```python
from build123d import *

# Parameters (mm, degrees)
EXTRUDE_1_DEPTH              = 5
SKETCH_2_R                   = 6.25
EXTRUDE_2_DEPTH              = 3
SKETCH_3_R                   = 5
EXTRUDE_3_DEPTH              = 5
HOLE_WIZARD_M4_1_D           = 4.5
HOLE_WIZARD_M4_1_CBORE_D     = 9
HOLE_WIZARD_M4_1_CBORE_DEPTH = 4
EXTRUDE_4_DEPTH              = 5
EXTRUDE_5_DEPTH              = 5
EXTRUDE_5_DEPTH_BACK         = 5
EXTRUDE_6_DEPTH              = 4.5
SKETCH_15_R                  = 10
CUT_EXTRUDE_2_DEPTH          = 20


with BuildPart() as part:
    # Sketch 1 → Extrude 1 (new body)
    with BuildSketch(Plane(origin=(0, 0, 0), x_dir=(1, 0, 0), z_dir=(0, 1, 0))):
        with BuildLine():
            Line((-15, 0), (-15, 60))
            ThreePointArc((-15, 60), (0, 75), (15, 60))
            Line((15, 60), (15, 0))
            ThreePointArc((15, 0), (0, -15), (-15, 0))
        make_face()
    extrude(amount=EXTRUDE_1_DEPTH)

    # Sketch 2 → Extrude 2 (add)
    with BuildSketch(Plane(origin=(0, 5, 0), x_dir=(1, 0, 0), z_dir=(0, 1, 0))):
        with Locations((0, 60)):
            Circle(SKETCH_2_R)
        Circle(SKETCH_2_R)
    extrude(amount=EXTRUDE_2_DEPTH)

    # Sketch 3 → Extrude 3 (add)
    with BuildSketch(Plane(origin=(0, 8, 0), x_dir=(1, 0, 0), z_dir=(0, 1, 0))):
        with Locations((0, 60)):
            Circle(SKETCH_3_R)
        Circle(SKETCH_3_R)
    extrude(amount=EXTRUDE_3_DEPTH)

    # Hole Wizard M4 _ _ _ _1 (through all)
    with Locations(Plane(origin=(0, 0, 0), x_dir=(-1, 0, 0), z_dir=(0, -1, 0))):
        with Locations((0, 60), (0, -25)):
            CounterBoreHole(HOLE_WIZARD_M4_1_D / 2, HOLE_WIZARD_M4_1_CBORE_D / 2, HOLE_WIZARD_M4_1_CBORE_DEPTH)

    # Sketch 8 → Extrude 4 (add)
    with BuildSketch(Plane.XZ):
        with BuildLine():
            Line((-5.13030215, 14.095389312), (23.060476474, 24.355993612))
            ThreePointArc((23.060476474, 24.355993612), (42.286167935, 15.39090645), (33.321080773, -3.834785012))
            Line((33.321080773, -3.834785012), (15, -10.503113073))
            Line((15, -10.503113073), (15, 0))
            ThreePointArc((15, 0), (8.603646545, 12.287280664), (-5.13030215, 14.095389312))
        make_face()
    extrude(amount=-EXTRUDE_4_DEPTH)

    # Sketch 9 → Extrude 5 (add, two sides)
    with BuildSketch(Plane.XZ) as extrude_5_sk:
        with BuildLine():
            Line((14.095389312, 5.13030215), (3.834785012, 33.321080773))
            Line((3.834785012, 33.321080773), (-1.295517138, 47.416470085))
            Line((-1.295517138, 47.416470085), (26.895261486, 57.677074385))
            Line((26.895261486, 57.677074385), (32.025563636, 43.581685073))
            Line((32.025563636, 43.581685073), (42.286167935, 15.39090645))
            ThreePointArc((42.286167935, 15.39090645), (33.321080773, -3.834785012), (14.095389312, 5.13030215))
        make_face()
    extrude(amount=EXTRUDE_5_DEPTH)
    extrude(extrude_5_sk.sketch, amount=-EXTRUDE_5_DEPTH_BACK)

    # Sketch 13 → Extrude 6 (add)
    with BuildSketch(Plane(origin=(0, 5, 0), x_dir=(1, 0, 0), z_dir=(0, 1, 0))):
        Polygon((37.155865785, -29.486295761), (26.895261486, -57.677074385), (-1.295517138, -47.416470085), (8.965087162, -19.225691462), align=None)
    extrude(amount=EXTRUDE_6_DEPTH)

    # Sketch 15 → Cut-Extrude 2 (cut)
    with BuildSketch(Plane(origin=(-15.39090645, 0, 42.286167935), x_dir=(0.939692621, 0, 0.342020143), z_dir=(-0.342020143, 0, 0.939692621))):
        with Locations((30, 10.5)):
            Circle(SKETCH_15_R)
    extrude(amount=-CUT_EXTRUDE_2_DEPTH, mode=Mode.SUBTRACT)


solid = part.part
```
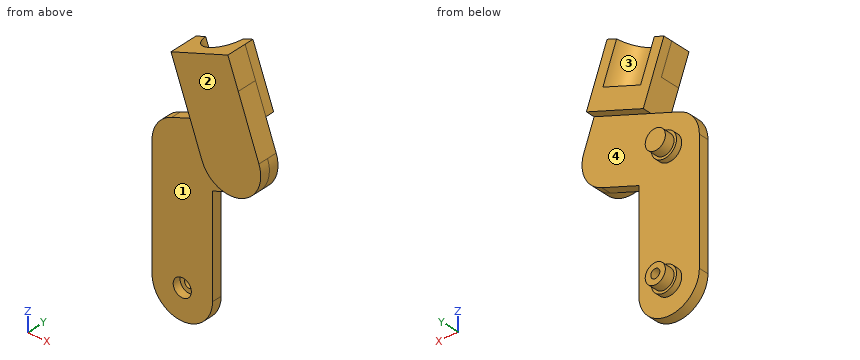
The model under review builds one solid part; all positions refer to its coordinate system, in mm. Face numbers are marked on the shaded views. A direction names the side the tool comes from. Coordinates: 2 decimals unless noted, no trailing zeros. Loops run counter-clockwise (first coordinate to the right, second up) from the corner with the lowest first, then second, coordinate; pieces in that order, holes last. Notation, with made-up numbers: (66.25, 43.25) -> (93.25, 43.25) arc R25 cw to (93.25, 66.25) -> close; hole circle Ø9 at (-5.5, 63). An arc over 180 degrees is marked (long way). Answer as CSV lines item,"result".
Item 1: For L1, parallel to X at y = 10.75, z = -60; L2, parallel to X at y = 2.45, z = -60; L3, parallel to Y at x = -10.5, z = 0, list the stretches that pass through material, from the lowest coordinate up.
Results below:
L1,"x = -5 to -2.25, 2.25 to 5"
L2,"x = -15 to -4.5, 4.5 to 15"
L3,"y = 0 to 5"
Item 2: Take a section at B-B, the plane x = 0. Count the separate pieces of the cut face and the enclosed holes in it, and give its area (3 significant figures).
Results below:
separate pieces,"3"
enclosed holes,"0"
area,"612 mm2"
Item 3: Draft analysis for pull direction X (two halves, no side actions). For the marked faces 3 and 4, state which applies: +X half, -X half, draft (parallel to the pull), parting line (faces both ways), or undercut.
Results below:
face 3,"undercut"
face 4,"draft"
Item 4: Insertion check: pin 1 (4 mm diameter, centred on y = 2, z = -36.5, fed in from +X); pin 2 (7 mm diameter, centred on x = 1.5, z = -59.5, fed in from -Y); pin 3 (3 mm diameter, centred on x = -7, z = -33.5, fed in from +Y); pin 4 (4 mm diameter, centred on x = 0, z = -60, fed in from -Y). Each pin has a flat end and moves straight along its axis. Give the tip position at first contact, or say it passes through.
Results below:
pin 1,"stops at x = 15"
pin 2,"stops at y = 0"
pin 3,"stops at y = 5"
pin 4,"passes through"
Item 5: Take a section at A-A, the plane y = 6.5. State the section outline as (x, z) points.
Results below:
outline,"circle Ø12.5 at (0, -60); circle Ø12.5 at (0, 0); (-1.3, 47.42) -> (8.97, 19.23) -> (37.16, 29.49) -> (26.9, 57.68) -> (21.41, 55.68) -> (28.25, 36.89) -> (11.03, 30.62) -> (4.19, 49.41) -> close; hole circle Ø4.5 at (0, -60)"
Item 6: Machinability: for the marked faces 1 and 2, which of the approach directions +Z, -Z, +X, -X, +Y, -Y give a long, thin tool a straight path to every point of the face, cutting with its end or side? Answer none if there is none.
Results below:
face 1,"-Z, -X, -Y"
face 2,"+Z, -Z, +X, -X, -Y"
Item 7: Take a section at C-C, the plane x = -8.5. State the section outline as (y, z) points.
Results below:
outline,"(0, -72.36) -> (5, -72.36) -> (5, 12.36) -> (0, 12.36) -> close"
